The listing builds one solid part. Answer for the finished solid, in the listing's coordinates (mm). Face numbers are marked on the shaded views. Give positions to 0.01 mm unless a question says otherwise; leave off trailing zeros. Order: outer loops, then holes, each group sorted by start corner. A loop starts at its lowest first (then second) coordinate and runs counter-clockwise, first axis right, second up. Notation, with made-up numbers: (22.5, -11.75) -> (46.5, -11.75) arc R33 ccw to (46.5, 22.25) -> close; hole circle Ø2 at (85.25, 76). An arc over 180 degrees is marked (long way). One line per question, with ' | ' between items. Start each with the question number.
Autodesk Inventor part; units mm, degrees
ref_plane "Work Plane1" through (-10.5, 0, 0) normal (1, 0, 0) x (0, 1, 0)
ref_plane "XZ Plane" through (0, 0, 0) normal (0, 1, 0) x (-1, 0, 0)
ref_plane "XY Plane" through (0, 0, 0) normal (0, 0, 1) x (1, 0, 0)
ref_plane "Work Plane1" through (-10.5, 0, 0) normal (1, 0, 0) x (0, 1, 0)
sketch "Sketch1" plane through (-10.5, 0, 0) normal (1, 0, 0) x (0, 1, 0)
  line L0 (5.5, 0) -> (-5.5, 0)
  line L1 (5.5, 4) -> (5.5, 0)
  line L2 (-5.5, 4) -> (-5.5, 0)
  line L3 (5.5, 4) -> (-5.5, 4)
extrude "Extrusion1" add sketch "Sketch1" along normal blind 21 draft 0
hole "Hole2" at (6.5, 0, 4) direction (0, 0, -1) diameter 4.5 depth 4
sketch "Sketch2" plane through (-10.5, -5.5, 4) normal (0, 0, 1) x (1, 0, 0)
  point P0 (17, 5.5)
hole "Hole1" at (-6.5, 0, 4) direction (0, 0, -1) diameter 4.5 depth 4
sketch "Sketch3" plane through (-10.5, -5.5, 4) normal (0, 0, 1) x (1, 0, 0)
  point P0 (4, 5.5)
properties part number "Y-axis Belt clamp" material "ASA Plastic"
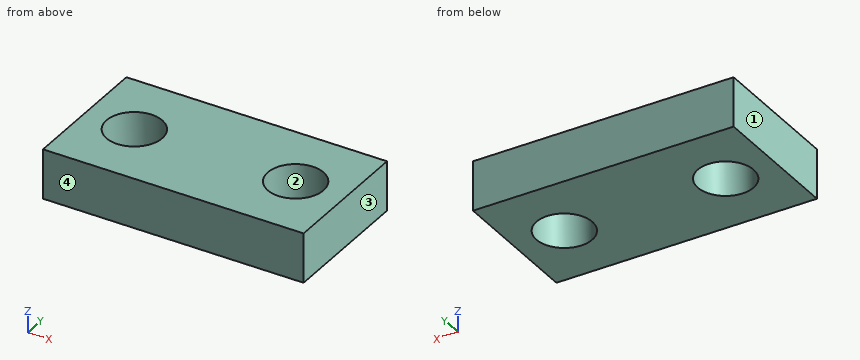
(1) Determine the mould class of the marked faces 1, 2, 3 and 4 for opening direction X: pulls with the +X half, pulls with the -X half, needs draft (parallel to the pull), parting line crosses it, or undercut.
(2) Consider line 1 (X direction, y = 0, z = 2.3); line 2 (X direction, y = -1.5, z = 1.8); line 3 (Y direction, x = 6.5, z = 1.25). Determine where each line is inside the solid, lowest interval first.
(3) The part is cut by section D-D on x = -4.5. Determine the outline of the cut face in (y, z).
(4) The part is cut by section A-A on y = 0. Determine the outline of the cut face in (x, z), plus the area to 3 significant figures.
(5) The part is cut by section C-C on x = 6.5. Determine the outline of the cut face in (y, z), plus the area to 3 significant figures.
(6) The part is cut by section B-B on z = 1.7. Determine the outline of the cut face in (x, y), plus the area to 3 significant figures.
(7) Given P1, Ø4, axis at x = -6.5, y = 0, coming from the +Z side; P2, Ø6, axis at x = 6.5, y = 0, coming from the -Z side, each flat-ended and moving along its own axis, determine where each tip first touches the part or whether it passes through.
Result sheet:
1) face 1: pulls with the -X half | face 2: undercut | face 3: pulls with the +X half | face 4: needs draft
2) line 1: x = -10.5 to -8.75, -4.25 to 4.25, 8.75 to 10.5 | line 2: x = -10.5 to -8.18, -4.82 to 4.82, 8.18 to 10.5 | line 3: y = -5.5 to -2.25, 2.25 to 5.5
3) outline: (-5.5, 0) -> (-1.03, 0) -> (-1.03, 4) -> (-5.5, 4) -> close; (1.03, 0) -> (5.5, 0) -> (5.5, 4) -> (1.03, 4) -> close
4) outline: (-10.5, 0) -> (-8.75, 0) -> (-8.75, 4) -> (-10.5, 4) -> close; (-4.25, 0) -> (4.25, 0) -> (4.25, 4) -> (-4.25, 4) -> close; (8.75, 0) -> (10.5, 0) -> (10.5, 4) -> (8.75, 4) -> close | area: 48.0 mm^2
5) outline: (-5.5, 0) -> (-2.25, 0) -> (-2.25, 4) -> (-5.5, 4) -> close; (2.25, 0) -> (5.5, 0) -> (5.5, 4) -> (2.25, 4) -> close | area: 26.0 mm^2
6) outline: (-10.5, -5.5) -> (10.5, -5.5) -> (10.5, 5.5) -> (-10.5, 5.5) -> close; hole circle Ø4.5 at (-6.5, 0); hole circle Ø4.5 at (6.5, 0) | area: 199 mm^2
7) P1: passes through | P2: stops at z = 0
